from build123d import *

# Parameters (mm, degrees)
SKETCH1_W           = 6.75
SKETCH1_H           = 5
BOSS_EXTRUDE1_DEPTH = 3
FILLET3_R           = 1
FILLET4_R           = 1
FILLET6_R           = 4


with BuildPart() as part:
    # Sketch1 → Boss-Extrude1 (new body)
    with BuildSketch(Plane.XY):
        with Locations((3.375, 52.5)):
            Rectangle(SKETCH1_W, SKETCH1_H)
        with BuildLine():
            Line((0, 50), (6.75, 50))
            Line((6.75, 50), (6.75, 40.02))
            Line((6.75, 40.02), (1.79, 40.02))
            Line((1.79, 40.02), (1.79, 44.518418243))
            Line((1.79, 44.518418243), (0, 44.518418243))
            Line((0, 44.518418243), (0, 40))
            ThreePointArc((0, 40), (-39.300483317, 7.44795348), (-14.635408574, -37.226399448))
            Line((-14.635408574, -37.226399448), (-7.59560281, -49.419700707))
            ThreePointArc((-7.59560281, -49.419700707), (-49.854714097, 3.808868904), (0, 50))
        make_face()
    extrude(amount=BOSS_EXTRUDE1_DEPTH)

    # Fillet3
    fillet3_edges = [part.edges().sort_by_distance(p)[0] for p in [
        (-7.59560281, -49.419700707, 1.5),
    ]]
    fillet(fillet3_edges, radius=FILLET3_R)

    # Fillet4
    fillet4_edges = [part.edges().sort_by_distance(p)[0] for p in [
        (-14.635408574, -37.226399448, 1.5),
    ]]
    fillet(fillet4_edges, radius=FILLET4_R)

    # Fillet6
    fillet6_edges = [part.edges().sort_by_distance(p)[0] for p in [
        (0, 50, 1.5),
    ]]
    fillet(fillet6_edges, radius=FILLET6_R)


solid = part.part
Source: CAD feature listing. Evaluate the final solid. Frame: model axes, mm. A direction names the side the tool comes from. Coordinates: 2 decimals unless noted, no trailing zeros. Loops run counter-clockwise (first coordinate to the right, second up) from the corner with the lowest first, then second, coordinate; pieces in that order, holes last. Notation, with made-up numbers: M 8,-16 L 52,-16 A6 ccw 52,-10 Z; hole C 56,68.25 d5. An arc over 180 degrees is marked long. Answer in a Markdown table with one row per item.
Q1. Section D-D on y = 17. Return the cut outline in (x, z), plus the area to 3 significant figures.
Answers below:
| item | result |
|---|---|
| outline | M -47.02,0 L -36.21,0 L -36.21,3 L -47.02,3 Z |
| area | 32.4 mm^2 |
Q2. Section A-A on z = 1.65. Return the cut outline in (x, y), plus the area to 3 significant figures.
Answers below:
| item | result |
|---|---|
| outline | M -14.95,-37.1 A40 cw 0,40 L 0,44.52 L 1.79,44.52 L 1.79,40.02 L 6.75,40.02 L 6.75,55 L 0,55 L 0,53.85 A4 cw -3.7,49.86 A50 ccw -9.73,-49.04 A1 ccw -8.67,-47.56 L -14.46,-37.53 A1 ccw Z |
| area | 1,400 mm^2 |
Q3. Set-up query: faces 5 (the flat face through (0, 42, 1)), 6 (the flat face through (4, 40.02, 1)), 7 (the cylindrical face through (-49.96, 2.04, 1.48)). Return all of +Z, -Z, +X, -X, +Y, -Y with unobstructed straight access to the full face (end or side cutting, diameter ignored); none if empty.
Answers below:
| item | result |
|---|---|
| face 5 | +Z, -Z, -Y |
| face 6 | +Z, -Z, +X, -Y |
| face 7 | +Z, -Z, -X |
Q4. Draft query along X for faces 1 (the cylindrical face through (-1.097, 51.099, 1.521)), 2 (the flat face through (1, 44.518, 1)), 3 (the flat face through (-11.605, -42.475, 1.479)), 4 (the flat face through (-39, 11, 3)). Return one class per face: pulls with the +X half, pulls with the -X half, needs draft (parallel to the pull), parting line crosses it, or undercut.
Answers below:
| item | result |
|---|---|
| face 1 | pulls with the -X half |
| face 2 | undercut |
| face 3 | pulls with the +X half |
| face 4 | needs draft |
Q5. Section B-B on x = -25.5. Return the cut outline in (y, z), plus the area to 3 significant figures.
Answers below:
| item | result |
|---|---|
| outline | M -43.01,0 L -30.82,0 L -30.82,3 L -43.01,3 Z; M 30.82,0 L 43.01,0 L 43.01,3 L 30.82,3 Z |
| area | 73.1 mm^2 |
Q6. Ray query, probe 1 along Y at (x, z) = (-31, 2.5); probe 2 along Y at (x, z) = (-18, 1.5); probe 3 along X at (y, z) = (8, 2.65). Return the intervals inside material, ascending. Write a range as from..to.
Answers below:
| item | result |
|---|---|
| probe 1 | y = -39.23..-25.28, 25.28..39.23 |
| probe 2 | y = -46.65..-35.72, 35.72..46.65 |
| probe 3 | x = -49.36..-39.19 |
Q7. First-contact query: pin 1 (1.5 mm diameter, centred on x = 4.5, z = 1, fed in from -Y); pin 2 (0.5 mm diameter, centred on x = 0.5, z = 1.5, fed in from -Y); pin 3 (1.5 mm diameter, centred on x = -6.5, z = 2.5, fed in from +Y); pin 4 (12 mm diameter, centred on x = -20.5, y = 26.5, fed in from -Z). Flat tips, straight axial feed; report the tip coordinate or a pass-through.
Answers below:
| item | result |
|---|---|
| pin 1 | stops at y = 40.02 |
| pin 2 | stops at y = 44.52 |
| pin 3 | stops at y = 49.67 |
| pin 4 | passes through |
Q8. Section C-C on x = -11. Return the cut outline in (y, z) (3 decimals).
Answers below:
| item | result |
|---|---|
| outline | M -48.775,0 L -43.523,0 L -43.523,3 L -48.775,3 Z; M 38.458,0 L 48.775,0 L 48.775,3 L 38.458,3 Z |
